Input: part model. Units: mm. Frame: model coordinates. A direction names the side the tool comes from. Round coordinates to 2 decimals unless told otherwise and drop trailing zeros. Loops run counter-clockwise (first coordinate to the right, second up) from the corner with the lowest first, then second, coordinate; pieces in that order, holes last.
(1) Line query: line 1 (Z direction, x = 12, y = 2); line 2 (X direction, y = 35, z = -28); line 3 (Z direction, x = 41, y = 65). Output: solid intervals per line, ascending.
(2) Draft query along Z for faces 1 (the face through (33, 23, -30)), 2 (the face through (0, 5, -23)), 3 (the face through (17.205, 4.548, -11.317)), 4 (the face through (36, 5, 0)). Return one class per face: released by +Z, released by -Z, zero draft, split by the parting line, or undercut.
(3) First-contact query: pin 1 Ø17 at (x, z) = (60, -12) entering from -Y; pin 2 Ø5 at (x, y) = (46.5, 34) entering from -Z; pin 3 Ø2.5 at (y, z) = (37.5, -28) entering from -X; pin 4 Ø10 at (x, y) = (52, 50) entering from +Z. Flat tips, straight axial feed; report the tip coordinate or a pass-through.
(4) Cut plane A-A, the plane x = 36. Output: boundary loops of the cut face in (y, z) (3 decimals).
(5) Cut plane B-B, the plane z = -24. Output: boundary loops of the cut face in (x, y), and give its area (3 significant figures).
(6) Cut plane C-C, the plane y = 36. Output: boundary loops of the cut face in (x, z), and give its area (3 significant figures).
(7) Access query for faces 5 (the face through (37.953, 74.872, -29.853)), 6 (the face through (21, 42, -26)), 7 (the face through (53, 10, -12)), 8 (the face through (31, 21, -16)), 9 (the face through (35, 6, -33)). Directions: +Z, -Z, +X, -X, +Y, -Y. A direction counts if a zero-diameter tool reaches every point of the face in a straight line with its end or side. Return the directions, or none.
from build123d import *

# Parameters (mm, degrees)
SKETCH1_W                         = 72
SKETCH1_H                         = 35
BOSS_EXTRUDE1_DEPTH               = 10
SKETCH3_W                         = 72
SKETCH3_H                         = 5
CUT_EXTRUDE1_DEPTH                = 4
BOSS_EXTRUDE2_DEPTH               = 8
SKETCH5_R                         = 15
BOSS_EXTRUDE3_DEPTH               = 5
M12X1_25_TAPPED_HOLE1_D           = 10.8
M12X1_25_TAPPED_HOLE1_CSINK_D     = 12.05
M12X1_25_TAPPED_HOLE1_CSINK_ANGLE = 90
FILLET1_R                         = 15
SKETCH9_W                         = 10
SKETCH9_H                         = 22
BOSS_EXTRUDE4_DEPTH               = 40
CUT_EXTRUDE2_DEPTH                = 40
FILLET2_R                         = 12
M12X1_5_TAPPED_HOLE1_D            = 10.5
M12X1_5_TAPPED_HOLE1_CSINK_D      = 12.05
M12X1_5_TAPPED_HOLE1_CSINK_ANGLE  = 90


with BuildPart() as part:
    # Sketch1 → Boss-Extrude1 (new body)
    with BuildSketch(Plane(origin=(0, 0, 0), x_dir=(1, 0, 0), z_dir=(0, 1, 0))):
        with Locations((36, 17.5)):
            Rectangle(SKETCH1_W, SKETCH1_H)
    extrude(amount=BOSS_EXTRUDE1_DEPTH)

    # Sketch3 → Cut-Extrude1 (cut)
    with BuildSketch(Plane(origin=(0, 10, 0), x_dir=(1, 0, 0), z_dir=(0, 1, 0))):
        with Locations((36, 32.5)):
            Rectangle(SKETCH3_W, SKETCH3_H)
    extrude(amount=-CUT_EXTRUDE1_DEPTH, mode=Mode.SUBTRACT)

    # Sketch4 → Boss-Extrude2 (add)
    with BuildSketch(Plane(origin=(0, 0, -30), x_dir=(-1, 0, 0), z_dir=(0, 0, -1))):
        with BuildLine():
            Line((-51, 10), (-21, 10))
            Line((-21, 10), (-21, 60))
            ThreePointArc((-21, 60), (-36, 75), (-51, 60))
            Line((-51, 60), (-51, 10))
        make_face()
    extrude(amount=-BOSS_EXTRUDE2_DEPTH)

    # Sketch5 → Boss-Extrude3 (add)
    with BuildSketch(Plane(origin=(0, 0, -30), x_dir=(-1, 0, 0), z_dir=(0, 0, -1))):
        with Locations((-36, 60)):
            Circle(SKETCH5_R)
    extrude(amount=BOSS_EXTRUDE3_DEPTH)

    # M12x1.25 Tapped Hole1 (through all)
    with Locations(Plane(origin=(36, 60, -35), x_dir=(-1, 0, 0), z_dir=(0, 0, -1))):
        with Locations((0, 0)):
            CounterSinkHole(M12X1_25_TAPPED_HOLE1_D / 2, M12X1_25_TAPPED_HOLE1_CSINK_D / 2, counter_sink_angle=M12X1_25_TAPPED_HOLE1_CSINK_ANGLE)

    # Fillet1
    fillet1_edges = [part.edges().sort_by_distance(p)[0] for p in [
        (21, 10, -26),
        (51, 10, -26),
    ]]
    fillet(fillet1_edges, radius=FILLET1_R)

    # Sketch9 → Boss-Extrude4 (add)
    with BuildSketch(Plane(origin=(0, 10, 0), x_dir=(1, 0, 0), z_dir=(0, 1, 0))):
        with Locations((36, 11)):
            Rectangle(SKETCH9_W, SKETCH9_H)
    extrude(amount=BOSS_EXTRUDE4_DEPTH)

    # Sketch10 → Cut-Extrude2 (cut)
    with BuildSketch(Plane(origin=(41, 0, 0), x_dir=(0, 0, -1), z_dir=(1, 0, 0))):
        Polygon((22, 50), (0, 10), (0, 50), align=None)
    extrude(amount=-CUT_EXTRUDE2_DEPTH, mode=Mode.SUBTRACT)

    # Fillet2
    fillet2_edges = [part.edges().sort_by_distance(p)[0] for p in [
        (0, 5, 0),
        (72, 5, 0),
    ]]
    fillet(fillet2_edges, radius=FILLET2_R)

    # M12x1.5 Tapped Hole1 (through all)
    with Locations(Plane(origin=(12, 10, -12), x_dir=(0, 0, 1), z_dir=(0, 1, 0))):
        with Locations((0, 0), (0, 48)):
            CounterSinkHole(M12X1_5_TAPPED_HOLE1_D / 2, M12X1_5_TAPPED_HOLE1_CSINK_D / 2, counter_sink_angle=M12X1_5_TAPPED_HOLE1_CSINK_ANGLE)


solid = part.part
Reported:
1. line 1: z = -35 to -17.25, -6.75 to 0
1. line 2: x = 21 to 51
1. line 3: z = -35 to -22
2. face 1: released by -Z
2. face 2: zero draft
2. face 3: undercut
2. face 4: released by +Z
3. pin 1: stops at y = 0
3. pin 2: stops at z = -30
3. pin 3: stops at x = 21
3. pin 4: stops at z = -22
4. outline: (0, -35) - (6, -35) - (6, -30) - (45, -30) - (45, -35) - (53.975, -35) - (54.6, -34.375) - (54.6, -22) - (50, -22) - (10, 0) - (0, 0) - close; (65.4, -34.375) - (66.025, -35) - (75, -35) - (75, -22) - (65.4, -22) - close
5. outline: (0, 0) - (72, 0) - (72, 10) - (66, 10) arc R15 cw to (51, 25) - (51, 60) arc R15 ccw to (21, 60) - (21, 25) arc R15 cw to (6, 10) - (0, 10) - close; hole circle Ø10.8 at (36, 60)
5. area: 2,580 mm2
6. outline: (21, -30) - (51, -30) - (51, -22) - (41, -22) - (41, -14.3) - (31, -14.3) - (31, -22) - (21, -22) - close
6. area: 317 mm2
7. face 5: -Z
7. face 6: +Z, -Z, -X, +Y
7. face 7: +Z, +X, +Y
7. face 8: +Z, -X, +Y
7. face 9: -Z, +X, -X
